Can you work these out from the model? Positions are in its coordinate system, mm. Face numbers are marked on the shaded views. A direction names the side the tool comes from. Round coordinates to 2 decimals unless told otherwise and drop trailing zeros. Write each loop counter-clockwise with the first axis right and the second up, starting at its lowest first coordinate (ties: lowest second). Pieces come first, ordered by that corner, then holes. Notation, with made-up numbers: M 29.25,-9.5 L 48.25,-9.5 A22 ccw 48.25,25.5 Z; hole C 35.5,-37 d8. An arc over 180 degrees is marked long. Answer in a Markdown table with one row per item. Add a question column.
(1) If I drill on probe 1 along Y at (x, z) = (0, 9) (3 decimals); probe 2 along X at (y, z) = (0, 11.5) (3 decimals); probe 3 along X at (y, z) = (-1.5, 8.5), over which ranges is the centre line in solid material (lowest first)?
(2) Suppose I cut it at A-A, the plane x = 0. Write out the boundary of the cut face in (y, z) (3 decimals).
(3) Suppose I cut it at C-C, the plane y = 0. Write out the boundary of the cut face in (x, z) (3 decimals).
(4) If we mould it in two halves opening along Y, with no side actions, what happens to the marked faces 1, 2 and 3? For each: released by +Y, released by -Y, zero draft, split by the parting line, or undercut.
(5) Suppose I cut it at B-B, the plane z = 15.5. Write out the boundary of the cut face in (x, y) (3 decimals).
(6) For the marked faces 4 and 5, which set-ups out of +Z, -Z, +X, -X, +Y, -Y let a thin tool reach every point of the face, with its end or its side?
(7) I'm going to push flat-ended pins straight in: pin 1 (5 mm diameter, centred on x = -4.5, y = 1, fed in from -Z); pin 2 (2 mm diameter, centred on x = 2, y = -1, fed in from +Z). Where does each tip first touch, or does it pass through?
from build123d import *

# Parameters (mm, degrees)
F0_W     = 13
F0_H     = 13
F1_DEPTH = 20.5
F3_DEPTH = 19
F4_R     = 1


with BuildPart() as f1:
    # F0 (on Top) → F1 (new body)
    with BuildSketch(Plane.XY):
        Rectangle(F0_W, F0_H)
    extrude(amount=F1_DEPTH)

    # F2 (on face) → F3 (cut)
    with BuildSketch(Plane.XY.offset(20.5)):
        with BuildLine():
            Line((3.824265, 2.125), (-3.824265, 2.125))
            ThreePointArc((-3.824265, 2.125), (0, -4.375), (3.824265, 2.125))
        make_face()
    extrude(amount=-F3_DEPTH, mode=Mode.SUBTRACT)

    # F4
    f4_edges = [f1.edges().sort_by_distance(p)[0] for p in [
        (-6.5, 6.5, 10.25),
        (-6.5, -6.5, 10.25),
        (6.5, -6.5, 10.25),
        (6.5, 6.5, 10.25),
        (0, 6.5, 0),
        (-6.5, 0, 0),
        (6.5, 0, 0),
        (0, -6.5, 0),
        (0, -6.5, 20.5),
        (6.5, 0, 20.5),
        (0, 6.5, 20.5),
        (-6.5, 0, 20.5),
    ]]
    fillet(f4_edges, radius=F4_R)


solid = f1.part
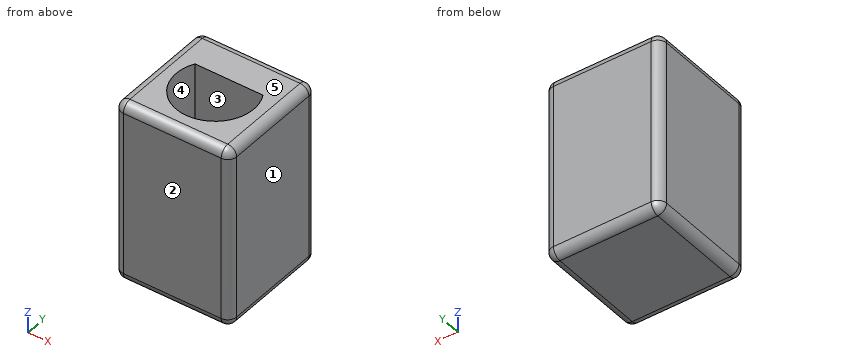
Calculated:
| question | item | result |
|---|---|---|
| 1 | probe 1 | -6.5 to -4.375, 2.125 to 6.5 |
| 1 | probe 2 | -6.5 to -4.375, 4.375 to 6.5 |
| 1 | probe 3 | -6.5 to -4.11, 4.11 to 6.5 |
| 2 | outline | M -6.5,1 A1 ccw -5.5,0 L 5.5,0 A1 ccw 6.5,1 L 6.5,19.5 A1 ccw 5.5,20.5 L 2.125,20.5 L 2.125,1.5 L -4.375,1.5 L -4.375,20.5 L -5.5,20.5 A1 ccw -6.5,19.5 Z |
| 3 | outline | M -6.5,1 A1 ccw -5.5,0 L 5.5,0 A1 ccw 6.5,1 L 6.5,19.5 A1 ccw 5.5,20.5 L 4.375,20.5 L 4.375,1.5 L -4.375,1.5 L -4.375,20.5 L -5.5,20.5 A1 ccw -6.5,19.5 Z |
| 4 | face 1 | zero draft |
| 4 | face 2 | released by -Y |
| 4 | face 3 | undercut |
| 5 | outline | M -6.5,-5.5 A1 ccw -5.5,-6.5 L 5.5,-6.5 A1 ccw 6.5,-5.5 L 6.5,5.5 A1 ccw 5.5,6.5 L -5.5,6.5 A1 ccw -6.5,5.5 Z; hole M -3.824,2.125 A4.375 ccw long 3.824,2.125 Z |
| 6 | face 4 | +Z |
| 6 | face 5 | +Z, +X, -X, +Y, -Y |
| 7 | pin 1 | z = 0 |
| 7 | pin 2 | z = 1.5 |
